from build123d import *

# Parameters (mm, degrees)
BOSS_EXTRUDE1_DEPTH     = 350
CUT_EXTRUDE1_DEPTH      = 531.758890646
CUT_EXTRUDE1_DEPTH_BACK = 531.758890646
SKETCH2_R               = 3
SKETCH3_R               = 11
SKETCH3_R_2             = 5
CUT_EXTRUDE2_DEPTH      = 515.987214376
SKETCH4_R               = 5
CUT_EXTRUDE3_DEPTH      = 525.030372184


with BuildPart() as part:
    # Sketch1 → Boss-Extrude1 (new body)
    with BuildSketch(Plane.XY):
        Polygon((3, 58.976984506), (3, -21.023015494), (57, -21.023015494), (57, 372.976984506), (63, 372.976984506), (63, -27.023015494), (57, -27.023015494), (-57, -27.023015494), (-57, -21.023015494), (-3, -21.023015494), (-3, 58.976984506), align=None)
    extrude(amount=BOSS_EXTRUDE1_DEPTH)

    # Sketch2 → Cut-Extrude1 (cut, two sides: drawn at the far end of the back side and taken through both)
    with BuildSketch(Plane(origin=(0, -21.023015494, 0), x_dir=(1, 0, 0), z_dir=(0, 1, 0)).offset(-CUT_EXTRUDE1_DEPTH_BACK)):
        with Locations((-30, -150)):
            Circle(SKETCH2_R)
        with Locations(Location((-30, -200, 0), (0, 0, 90))):
            Circle(SKETCH2_R)
        with Locations(Location((30, -200, 0), (0, 0, 90))):
            Circle(SKETCH2_R)
        with Locations(Location((30, -150, 0), (0, 0, 90))):
            Circle(SKETCH2_R)
    extrude(amount=CUT_EXTRUDE1_DEPTH + CUT_EXTRUDE1_DEPTH_BACK, mode=Mode.SUBTRACT)

    # Sketch3 → Cut-Extrude2 (cut, through all)
    with BuildSketch(Plane(origin=(3, 0, 0), x_dir=(0, 0, -1), z_dir=(1, 0, 0))):
        with Locations(Location((-175, 18.976984506, 0), (0, 0, 90))):
            Circle(SKETCH3_R)
        with Locations(Location((-301.895890035, 18.976984506, 0), (0, 0, 90))):
            Circle(SKETCH3_R_2)
        with Locations(Location((-48.104109965, 18.976984506, 0), (0, 0, 90))):
            Circle(SKETCH3_R_2)
    extrude(amount=-CUT_EXTRUDE2_DEPTH, mode=Mode.SUBTRACT)

    # Sketch4 → Cut-Extrude3 (cut, through all)
    with BuildSketch(Plane.ZY.offset(-57)):
        with Locations((48.1, 272.976984506)):
            Circle(SKETCH4_R)
        with Locations(Location((301.9, 272.976984506, 0), (0, 0, 180))):
            Circle(SKETCH4_R)
    extrude(amount=-CUT_EXTRUDE3_DEPTH, mode=Mode.SUBTRACT)


solid = part.part
The listing builds one solid part. Answer for the finished solid, in the listing's coordinates (mm). A direction names the side the tool comes from. Round coordinates to 2 decimals unless told otherwise and drop trailing zeros. Order: outer loops, then holes, each group sorted by start corner. A loop starts at its lowest first (then second) coordinate and runs counter-clockwise, first axis right, second up. Notation, with made-up numbers: (2.25, -30) -> (54.25, -30) arc R20 cw to (54.25, -13) -> close; hole circle Ø8 at (44.25, -36.5). An arc over 180 degrees is marked (long way). One line per item, written item: value.
Item 1: Find section C-C, the plane x = 50. Give the vertices of the cut face in (y, z).
Taken from the geometry:
outline: (-27.02, 0) -> (-21.02, 0) -> (-21.02, 350) -> (-27.02, 350) -> close
Item 2: For faces 5 (the flat face through (3, 2, 173)), 6 (the cylindrical face through (0.042, 21.284, 43.668)), 7 (the flat face through (-3, 1, 173)), 8 (the flat face through (63, 176, 173)), determine the directions among +Z, -Z, +X, -X, +Y, -Y from which every point of the face is accessible in a straight line to the end or side of a thin tool.
Taken from the geometry:
face 5: +Z, -Z, +Y
face 6: -X
face 7: +Z, -Z, -X, +Y
face 8: +Z, -Z, +X, +Y, -Y
Item 3: Given P1, Ø9.5, axis at x = -30, z = 150, coming from the +Y side; P2, Ø8, axis at x = 30, z = 200, coming from the -Y side; P3, Ø6, axis at y = 18.98, z = 301.9, coming from the -X side; P4, Ø24, axis at y = 33.5, z = 256.5, coming from the -X side, each flat-ended and moving along its own axis, determine where each tip first touches the part or whether it passes through.
Taken from the geometry:
P1: stops at y = -21.02
P2: stops at y = -27.02
P3: stops at x = 57
P4: stops at x = -3
Item 4: Find section A-A, the plane y = 41. Give the vertices of the cut face in (x, z), then the cut area to 3 significant figures.
Taken from the geometry:
outline: (-3, 0) -> (3, 0) -> (3, 350) -> (-3, 350) -> close; (57, 0) -> (63, 0) -> (63, 350) -> (57, 350) -> close
area: 4,200 mm2
Item 5: For a pull along Z with two mould halves and no side action, classify faces 1 (the flat face through (61, 144, 350)), 2 (the flat face through (61, 144, 0)), 3 (the cylindrical face through (0.04, 21.28, 297.46)), 4 (the flat face through (-30, -21.023, 173)) as released by +Z, released by -Z, zero draft, split by the parting line, or undercut.
Taken from the geometry:
face 1: released by +Z
face 2: released by -Z
face 3: undercut
face 4: zero draft
Item 6: Find section D-D, the plane y = 336. Give the vertices of the cut face in (x, z).
Taken from the geometry:
outline: (57, 0) -> (63, 0) -> (63, 350) -> (57, 350) -> close
Item 7: Find section B-B, the plane z = 34. Give the vertices of the cut face in (x, y), then the cut area to 3 significant figures.
Taken from the geometry:
outline: (-57, -27.02) -> (63, -27.02) -> (63, 372.98) -> (57, 372.98) -> (57, -21.02) -> (3, -21.02) -> (3, 58.98) -> (-3, 58.98) -> (-3, -21.02) -> (-57, -21.02) -> close
area: 3,560 mm2
Item 8: Straight lines are drawn through the part: L1, parallel to X at y = -22.85, z = 150; L2, parallel to X at y = 7.5, z = 54.5; L3, parallel to Y at x = 61.7, z = 301.9. For each, find the intervals that lie inside material, in ascending order.
Taken from the geometry:
L1: x = -57 to -33, -27 to 27, 33 to 63
L2: x = -3 to 3, 57 to 63
L3: y = -27.02 to 267.98, 277.98 to 372.98
